from build123d import *

# Parameters (mm, degrees)
SKETCH1_W                                        = 150
SKETCH1_H                                        = 40
BOSS_EXTRUDE1_DEPTH                              = 10
BOSS_EXTRUDE2_DEPTH                              = 10
CBORE_FOR_1_4_SOCKET_HEAD_CAP_SCREW1_D           = 6.7564
CBORE_FOR_1_4_SOCKET_HEAD_CAP_SCREW1_CBORE_D     = 11.1125
CBORE_FOR_1_4_SOCKET_HEAD_CAP_SCREW1_CBORE_DEPTH = 6.35
FILLET1_R                                        = 6
FILLET2_R                                        = 3
FILLET3_R                                        = 1
SHELL4_START                                     = -14
SHELL4_OUTLINE_W                                 = 146
SHELL4_OUTLINE_H                                 = 8
SHELL4_DEPTH                                     = 28
SHELL4_START_2                                   = 12
SHELL4_2_OUTLINE_R                               = 7.55625
SHELL4_2_DEPTH                                   = 6
SHELL4_3_DEPTH                                   = 8


with BuildPart() as part:
    # Sketch1 → Boss-Extrude1 (new body)
    with BuildSketch(Plane(origin=(0, 0, 0), x_dir=(1, 0, 0), z_dir=(0, 1, 0))):
        Rectangle(SKETCH1_W, SKETCH1_H)
    extrude(amount=BOSS_EXTRUDE1_DEPTH)

    # Sketch2 → Boss-Extrude2 (add)
    with BuildSketch(Plane.XY.offset(20)):
        with BuildLine():
            Line((-45, 0), (-5, 0))
            Line((-5, 0), (-5, 65))
            ThreePointArc((-5, 65), (-25, 85), (-45, 65))
            Line((-45, 65), (-45, 0))
        make_face()
    extrude(amount=-BOSS_EXTRUDE2_DEPTH)

    # CBORE for 1/4 Socket Head Cap Screw1 (through all)
    with Locations(Plane.XY.offset(20)):
        with Locations((-25, 65)):
            CounterBoreHole(CBORE_FOR_1_4_SOCKET_HEAD_CAP_SCREW1_D / 2, CBORE_FOR_1_4_SOCKET_HEAD_CAP_SCREW1_CBORE_D / 2, CBORE_FOR_1_4_SOCKET_HEAD_CAP_SCREW1_CBORE_DEPTH)

    # Fillet1
    fillet1_edges = [part.edges().sort_by_distance(p)[0] for p in [
        (-75, 5, -20),
        (75, 5, -20),
        (75, 5, 20),
        (-75, 5, 20),
    ]]
    fillet(fillet1_edges, radius=FILLET1_R)

    # Fillet2
    fillet2_edges = [part.edges().sort_by_distance(p)[0] for p in [
        (-45, 10, 15),
        (-5, 10, 15),
    ]]
    fillet(fillet2_edges, radius=FILLET2_R)

    # Fillet3
    fillet3_edges = [part.edges().sort_by_distance(p)[0] for p in [
        (-45, 39, 10),
        (-25, 85, 10),
        (-45, 39, 20),
        (-25, 85, 20),
        (0, 10, -20),
        (75, 10, 0),
        (-75, 10, 0),
        (-58.5, 10, 20),
        (73.242640687, 10, 18.242640687),
        (-73.242640687, 10, 18.242640687),
        (-73.242640687, 10, -18.242640687),
        (73.242640687, 10, -18.242640687),
        (33.5, 10, 20),
        (-5, 39, 20),
        (-5, 39, 10),
        (-45.878679656, 10.878679656, 20),
        (-45.878679656, 10.878679656, 10),
        (-4.121320344, 10.878679656, 10),
        (-4.121320344, 10.878679656, 20),
    ]]
    fillet(fillet3_edges, radius=FILLET3_R)

    # Shell4: read off the stored shape, not the designer's step
    # Shell4 outline → Shell4 (cut)
    with BuildSketch(Plane.XY.offset(SHELL4_START)):
        with Locations((0, 4)):
            Rectangle(SHELL4_OUTLINE_W, SHELL4_OUTLINE_H)
    extrude(amount=SHELL4_DEPTH, mode=Mode.SUBTRACT)

    # Shell4 2 outline → Shell4 2 (cut)
    with BuildSketch(Plane.XY.offset(SHELL4_START_2)):
        with BuildLine():
            ThreePointArc((-43, 13), (-44.464466094, 9.464466094), (-48, 8))
            Line((-48, 8), (-2, 8))
            ThreePointArc((-2, 8), (-5.535533906, 9.464466094), (-7, 13))
            Line((-7, 13), (-7, 65))
            ThreePointArc((-7, 65), (-25, 83), (-43, 65))
            Line((-43, 65), (-43, 13))
        make_face()
        with Locations((-25, 65)):
            Circle(SHELL4_2_OUTLINE_R, mode=Mode.SUBTRACT)
    extrude(amount=SHELL4_2_DEPTH, mode=Mode.SUBTRACT)

    # Shell4 3 outline → Shell4 3 (cut)
    with BuildSketch(Plane(origin=(0, 0, 0), x_dir=(1, 0, 0), z_dir=(0, 1, 0))):
        with BuildLine():
            Line((-69, -18), (69, -18))
            ThreePointArc((69, -18), (71.828427125, -16.828427125), (73, -14))
            Line((73, -14), (-73, -14))
            ThreePointArc((-73, -14), (-71.828427125, -16.828427125), (-69, -18))
        make_face()
        with BuildLine():
            Line((69, 18), (-69, 18))
            ThreePointArc((-69, 18), (-71.828427125, 16.828427125), (-73, 14))
            Line((-73, 14), (73, 14))
            ThreePointArc((73, 14), (71.828427125, 16.828427125), (69, 18))
        make_face()
    extrude(amount=SHELL4_3_DEPTH, mode=Mode.SUBTRACT)


solid = part.part
Verification items for the finished model (mm, model axes). A direction names the side the tool comes from. Round coordinates to 2 decimals unless told otherwise and drop trailing zeros. Write each loop counter-clockwise with the first axis right and the second up, starting at its lowest first coordinate (ties: lowest second). Pieces come first, ordered by that corner, then holes.
(1) Section check D-D (x = 19). Enter the section's corners in (y, z), plus the area to 3 significant figures.
Returned:
outline: (0, -20) - (9, -20) arc R1 ccw to (10, -19) - (10, 19) arc R1 ccw to (9, 20) - (0, 20) - (0, 18) - (8, 18) - (8, -18) - (0, -18) - close
area: 112 mm2
(2) Section check B-B (y = 33.5). Enter the section's corners in (x, z), plus the area to 3 significant figures.
Returned:
outline: (-45, 11) arc R1 ccw to (-44, 10) - (-6, 10) arc R1 ccw to (-5, 11) - (-5, 19) arc R1 ccw to (-6, 20) - (-44, 20) arc R1 ccw to (-45, 19) - close; hole (-43, 12) - (-7, 12) - (-7, 18) - (-43, 18) - close
area: 183 mm2
(3) Section check A-A (x = -25). Enter the section's corners in (y, z).
Returned:
outline: (0, -20) - (9, -20) arc R1 ccw to (10, -19) - (10, 10) - (61.62, 10) - (61.62, 13.65) - (59.44, 13.65) - (59.44, 20) - (0, 20) - (0, 18) - (57.44, 18) - (57.44, 12) - (8, 12) - (8, -18) - (0, -18) - close; (68.38, 10) - (84, 10) arc R1 ccw to (85, 11) - (85, 19) arc R1 ccw to (84, 20) - (70.56, 20) - (70.56, 13.65) - (68.38, 13.65) - close; hole (72.56, 12) - (83, 12) - (83, 18) - (72.56, 18) - close
(4) Access from +Z, -Z, +X, -X, +Y, -Y to the whole of each face (thin tool, end or side, straight path). Record for faces 5 (the cylindrical face through (73.289, 4.563, -18.196)), 6 (the cylindrical face through (-22.44, 60.07, 16.87)), 7 (the cylindrical face through (-5, 9, 15)).
Returned:
face 5: -Z, +X, +Y, -Y
face 6: +Z
face 7: -Y
(5) Section check C-C (z = 0.5). Enter the section's corners in (x, y).
Returned:
outline: (-75, 0) - (-73, 0) - (-73, 8) - (73, 8) - (73, 0) - (75, 0) - (75, 9) arc R1 ccw to (74, 10) - (-74, 10) arc R1 ccw to (-75, 9) - close
(6) Material ranges on line 1 (Y direction, x = -25, z = 11.1); line 2 (Y direction, x = -25, z = 18.75); line 3 (Y direction, x = -25, z = 16), recorded low to high.
Returned:
line 1: y = 8 to 61.62, 68.38 to 85
line 2: y = 0 to 59.44, 70.56 to 85
line 3: y = 57.44 to 59.44, 70.56 to 72.56, 83 to 85
(7) Depth check by flat-ended pin: pin 1 Ø2 at (x, z) = (-4, -0.5) entering from -Y; pin 2 Ø12 at (y, z) = (18, 11) entering from -X; pin 3 Ø12 at (x, y) = (-2.5, 51.5) entering from +Z; pin 4 Ø6.5 at (y, z) = (31.5, 15) entering from +X. Enter the tip coordinate at first touch or a pass-through.
Returned:
pin 1: stops at y = 8
pin 2: stops at x = -45.17
pin 3: stops at z = 20
pin 4: stops at x = -5
(8) Mould release check, pull along X, two halves, no side actions. Record for faces 1 (the flat face through (0, 0, -19)), 2 (the cylindrical face through (-71.859, 3.944, 16.797)), 3 (the cylindrical face through (-73.196, 4.563, 18.289)), 4 (the cylindrical face through (73.196, 4.563, 18.289)): pulls with the +X half, pulls with the -X half, needs draft (parallel to the pull), parting line crosses it, or undercut.
Returned:
face 1: needs draft
face 2: undercut
face 3: pulls with the -X half
face 4: pulls with the +X half
